Autodesk Fusion 360 part; units mm, degrees
sketch "Sketch1" plane through (0, 0, 0) normal (0, 1, 0) x (1, 0, 0)
  line L0 (0, 0) -> (85, 0)
  line L1 (85, 0) -> (85, 65)
  line L2 (85, 65) -> (0, 65)
  line L3 (0, 65) -> (0, 0)
  line L4 (0, 17.25) -> (63, 17.25) construction
  line L5 (63, 17.25) -> (63, 0) construction
  line L6 (63, 17.25) -> (63, 65) construction
  line L7 (63, 17.25) -> (63, 54.75)
  circle A0 centre (63, 17.25) radius 11
  circle A1 centre (63, 54.75) radius 4
  line L8 (63, 6.25) -> (63, 0)
  dimension "d1" = 85
  dimension "d2" = 65
  dimension "d4" = 63
  dimension "d5" = 37.5
  dimension "d6" = 22
  dimension "d7" = 8
  dimension "d9" = 6.25
extrude "Extrude1" add sketch "Sketch1" along normal blind 7.5
fillet "Fillet1" radius 5 1 edges at (85, 3.75, 0)
fillet "Fillet2" radius 5 1 edges at (85, 3.75, -65)
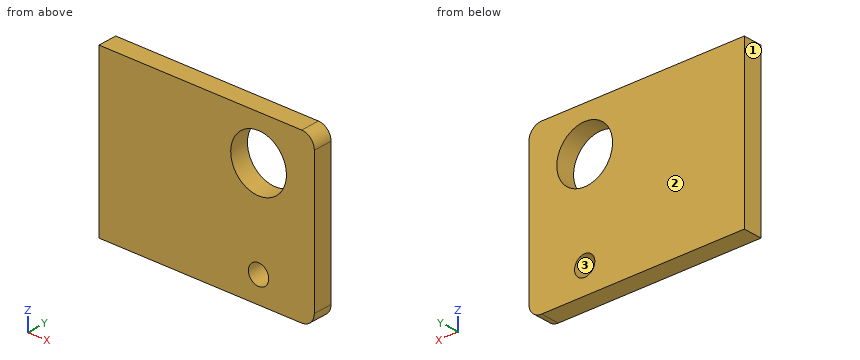
CAD build for the part. Positions are in the model's coordinates, mm. Face numbers are marked on the shaded views. Coordinates: 2 decimals unless noted, no trailing zeros. Order: outer loops, then holes, each group sorted by start corner. A loop starts at its lowest first (then second) coordinate and runs counter-clockwise, first axis right, second up.
Item 1: Band-saw the part on B-B on x = 63. List the corners of the cut face in (y, z), plus the area to 4 significant figures.
Check sheet entries:
outline: (0, -65) - (7.5, -65) - (7.5, -58.75) - (0, -58.75) - close; (0, -50.75) - (7.5, -50.75) - (7.5, -28.25) - (0, -28.25) - close; (0, -6.25) - (7.5, -6.25) - (7.5, 0) - (0, 0) - close
area: 262.5 mm2
Item 2: Two-plate mould, pull along X, no slides. Class the marked faces 1, 2 and 3: +X half, -X half, draft (parallel to the pull), parting line (faces both ways), or undercut.
Check sheet entries:
face 1: -X half
face 2: draft
face 3: undercut
Item 3: Band-saw the part on A-A on z = -54.75. List the corners of the cut face in (x, y), plus the area to 4 significant figures.
Check sheet entries:
outline: (0, 0) - (59, 0) - (59, 7.5) - (0, 7.5) - close; (67, 0) - (85, 0) - (85, 7.5) - (67, 7.5) - close
area: 577.5 mm2
Item 4: Band-saw the part on C-C on y = 3. List the corners of the cut face in (x, z), plus the area to 3 significant figures.
Check sheet entries:
outline: (0, -65) - (80, -65) arc R5 ccw to (85, -60) - (85, -5) arc R5 ccw to (80, 0) - (0, 0) - close; hole circle Ø22 at (63, -17.25); hole circle Ø8 at (63, -54.75)
area: 5,080 mm2
Item 5: Pin check, flat tip, straight feed: pin 1 Ø17.5 at (x, z) = (63, -17.25) entering from -Y. Stop position of the tip, or through.
Check sheet entries:
pin 1: passes through
Item 6: Band-saw the part on D-D on z = -17.25. List the corners of the cut face in (x, y).
Check sheet entries:
outline: (0, 0) - (52, 0) - (52, 7.5) - (0, 7.5) - close; (74, 0) - (85, 0) - (85, 7.5) - (74, 7.5) - close
Item 7: Drill centre lines: L1, parallel to Z at x = 63, y = 3.25; L2, parallel to X at y = 4.5, z = -54.75; L3, parallel to X at y = 5.75, z = -23. Where is each one in solid material? Low to high.
Check sheet entries:
L1: z = -65 to -58.75, -50.75 to -28.25, -6.25 to 0
L2: x = 0 to 59, 67 to 85
L3: x = 0 to 53.62, 72.38 to 85
